```python
from build123d import *

# Parameters (mm, degrees)
BOSS_EXTRUDE1_DEPTH = 6.6


with BuildPart() as part:
    # Model → Boss-Extrude1 (new body)
    with BuildSketch(Plane.XY):
        with BuildLine():
            Line((72.9, 1.275), (72.9, -1.275))
            ThreePointArc((72.9, -1.275), (73.046446609, -1.628553391), (73.4, -1.775))
            Line((73.4, -1.775), (77.9, -1.775))
            Line((77.9, -1.775), (77.9, -3.36))
            ThreePointArc((77.9, -3.36), (78.046446609, -3.713553391), (78.4, -3.86))
            Line((78.4, -3.86), (82.4, -3.86))
            ThreePointArc((82.4, -3.86), (82.753553391, -3.713553391), (82.9, -3.36))
            Line((82.9, -3.36), (82.9, -1.775))
            Line((82.9, -1.775), (93.9, -1.775))
            Line((93.9, -1.775), (93.9, -27.3))
            Line((93.9, -27.3), (97.9, -27.3))
            ThreePointArc((97.9, -27.3), (99.667766953, -28.032233047), (100.4, -29.8))
            Line((100.4, -29.8), (100.4, -39.8))
            ThreePointArc((100.4, -39.8), (99.667766953, -41.567766953), (97.9, -42.3))
            Line((97.9, -42.3), (93.9, -42.3))
            Line((93.9, -42.3), (93.9, -55))
            Line((93.9, -55), (-93.9, -55))
            Line((-93.9, -55), (-93.9, -42.3))
            Line((-93.9, -42.3), (-97.9, -42.3))
            ThreePointArc((-97.9, -42.3), (-99.667766953, -41.567766953), (-100.4, -39.8))
            Line((-100.4, -39.8), (-100.4, -29.8))
            ThreePointArc((-100.4, -29.8), (-99.667766953, -28.032233047), (-97.9, -27.3))
            Line((-97.9, -27.3), (-93.9, -27.3))
            Line((-93.9, -27.3), (-93.9, -1.775))
            Line((-93.9, -1.775), (-82.9, -1.775))
            Line((-82.9, -1.775), (-82.9, -3.36))
            ThreePointArc((-82.9, -3.36), (-82.753553391, -3.713553391), (-82.4, -3.86))
            Line((-82.4, -3.86), (-78.4, -3.86))
            ThreePointArc((-78.4, -3.86), (-78.046446609, -3.713553391), (-77.9, -3.36))
            Line((-77.9, -3.36), (-77.9, -1.775))
            Line((-77.9, -1.775), (-73.4, -1.775))
            ThreePointArc((-73.4, -1.775), (-73.046446609, -1.628553391), (-72.9, -1.275))
            Line((-72.9, -1.275), (-72.9, 1.275))
            ThreePointArc((-72.9, 1.275), (-73.046446609, 1.628553391), (-73.4, 1.775))
            Line((-73.4, 1.775), (-77.9, 1.775))
            Line((-77.9, 1.775), (-77.9, 3.36))
            ThreePointArc((-77.9, 3.36), (-78.046446609, 3.713553391), (-78.4, 3.86))
            Line((-78.4, 3.86), (-82.4, 3.86))
            ThreePointArc((-82.4, 3.86), (-82.753553391, 3.713553391), (-82.9, 3.36))
            Line((-82.9, 3.36), (-82.9, 1.775))
            Line((-82.9, 1.775), (-93.9, 1.775))
            Line((-93.9, 1.775), (-93.9, 27.3))
            Line((-93.9, 27.3), (-97.9, 27.3))
            ThreePointArc((-97.9, 27.3), (-99.667766953, 28.032233047), (-100.4, 29.8))
            Line((-100.4, 29.8), (-100.4, 39.8))
            ThreePointArc((-100.4, 39.8), (-99.667766953, 41.567766953), (-97.9, 42.3))
            Line((-97.9, 42.3), (-93.9, 42.3))
            Line((-93.9, 42.3), (-93.9, 55))
            Line((-93.9, 55), (93.9, 55))
            Line((93.9, 55), (93.9, 42.3))
            Line((93.9, 42.3), (97.9, 42.3))
            ThreePointArc((97.9, 42.3), (99.667766953, 41.567766953), (100.4, 39.8))
            Line((100.4, 39.8), (100.4, 29.8))
            ThreePointArc((100.4, 29.8), (99.667766953, 28.032233047), (97.9, 27.3))
            Line((97.9, 27.3), (93.9, 27.3))
            Line((93.9, 27.3), (93.9, 1.775))
            Line((93.9, 1.775), (82.9, 1.775))
            Line((82.9, 1.775), (82.9, 3.36))
            ThreePointArc((82.9, 3.36), (82.753553391, 3.713553391), (82.4, 3.86))
            Line((82.4, 3.86), (78.4, 3.86))
            ThreePointArc((78.4, 3.86), (78.046446609, 3.713553391), (77.9, 3.36))
            Line((77.9, 3.36), (77.9, 1.775))
            Line((77.9, 1.775), (73.4, 1.775))
            ThreePointArc((73.4, 1.775), (73.046446609, 1.628553391), (72.9, 1.275))
        make_face()
        with BuildLine():
            Line((29.75, 34.05), (29.75, -29.45))
            ThreePointArc((29.75, -29.45), (26.25, -32.95), (22.75, -29.45))
            Line((22.75, -29.45), (22.75, 34.05))
            ThreePointArc((22.75, 34.05), (26.25, 37.55), (29.75, 34.05))
        make_face(mode=Mode.SUBTRACT)
        with BuildLine():
            Line((-29.75, 34.05), (-29.75, -29.45))
            ThreePointArc((-29.75, -29.45), (-26.25, -32.95), (-22.75, -29.45))
            Line((-22.75, -29.45), (-22.75, 34.05))
            ThreePointArc((-22.75, 34.05), (-26.25, 37.55), (-29.75, 34.05))
        make_face(mode=Mode.SUBTRACT)
        with BuildLine():
            Line((2.54, -29.45), (2.54, 34.05))
            ThreePointArc((2.54, 34.05), (0, 36.59), (-2.54, 34.05))
            Line((-2.54, 34.05), (-2.54, -29.45))
            ThreePointArc((-2.54, -29.45), (0, -31.99), (2.54, -29.45))
        make_face(mode=Mode.SUBTRACT)
        with BuildLine():
            Line((-39.75, -35), (-39.75, 35))
            ThreePointArc((-39.75, 35), (-42.678932188, 42.071067812), (-49.75, 45))
            Line((-49.75, 45), (-52.9, 45))
            ThreePointArc((-52.9, 45), (-59.971067812, 42.071067812), (-62.9, 35))
            Line((-62.9, 35), (-62.9, -35))
            ThreePointArc((-62.9, -35), (-59.971067812, -42.071067812), (-52.9, -45))
            Line((-52.9, -45), (-49.75, -45))
            ThreePointArc((-49.75, -45), (-42.678932188, -42.071067812), (-39.75, -35))
        make_face(mode=Mode.SUBTRACT)
        with BuildLine():
            Line((62.9, -35), (62.9, 35))
            ThreePointArc((62.9, 35), (59.971067812, 42.071067812), (52.9, 45))
            Line((52.9, 45), (49.75, 45))
            ThreePointArc((49.75, 45), (42.678932188, 42.071067812), (39.75, 35))
            Line((39.75, 35), (39.75, -35))
            ThreePointArc((39.75, -35), (42.678932188, -42.071067812), (49.75, -45))
            Line((49.75, -45), (52.9, -45))
            ThreePointArc((52.9, -45), (59.971067812, -42.071067812), (62.9, -35))
        make_face(mode=Mode.SUBTRACT)
    extrude(amount=BOSS_EXTRUDE1_DEPTH)


solid = part.part
```
Part model, mm, in its own coordinate system. A direction names the side the tool comes from. Round coordinates to 2 decimals unless told otherwise and drop trailing zeros. Loops run counter-clockwise (first coordinate to the right, second up) from the corner with the lowest first, then second, coordinate; pieces in that order, holes last.
Item 1: Drill centre lines: line 1 (X direction, y = 5.5, z = 1); line 2 (X direction, y = -35, z = 4.75); line 3 (X direction, y = -43, z = 2.75). Where is each one in solid material? Low to high.
Item 2: Drop flat-ended pins along their axis: P1, Ø3, axis at y = 0.5, z = 2.5, coming from the -X side; P2, Ø3.5, axis at y = -13, z = 3.5, coming from the +X side; P3, Ø3, axis at x = 95.5, z = 3, coming from the -Y side. Give the stop position or say it passes through.
Item 3: Mould opens along X. For faces 5 (the face through (96, 27.3, 3)), 6 (the face through (-26.33, -32.95, 3.25)), 7 (the face through (-93.9, 49, 3)) say: +X half, -X half, draft (parallel to the pull), parting line (faces both ways), or undercut.
Item 4: Cut at D-D, the plane z = 1. State how many separate pieces and enclosed holes the cut face has, then the cut area to 3 significant figures.
Item 5: Cut at B-B, the plane y = -8.5. Give the cut face in (x, z), then the cut area to 3 significant figures.
Item 6: Cut at A-A, the plane x = -87. Give the cut face in (y, z) (3 decimals), then the cut area to 3 significant figures.
Item 7: Cut at C-C, the plane x = 26.25. Give the cut face in (y, z).
Item 8: 3-axis set-ups, long thin cutter, end or side, ignore diameter. For faces 1 (the face through (-93.9, 14, 3)), 2 (the face through (93.9, 15, 3)), 3 (the face through (93.9, 49, 3)), 4 (the face through (22.75, 2, 3)): which of +Z, -Z, +X, -X, +Y, -Y reach the whole face in a straight line?
A:
1. line 1: x = -93.9 to -62.9, -39.75 to -29.75, -22.75 to -2.54, 2.54 to 22.75, 29.75 to 39.75, 62.9 to 93.9
1. line 2: x = -100.4 to -62.9, -39.75 to 39.75, 62.9 to 100.4
1. line 3: x = -93.9 to -58.9, -43.75 to 43.75, 58.9 to 93.9
2. P1: stops at x = -93.9
2. P2: stops at x = 93.9
2. P3: stops at y = -42.3
3. face 5: draft
3. face 6: undercut
3. face 7: -X half
4. separate pieces: 1
4. enclosed holes: 5
4. area: 15,500 mm2
5. outline: (-93.9, 0) - (-62.9, 0) - (-62.9, 6.6) - (-93.9, 6.6) - close; (-39.75, 0) - (-29.75, 0) - (-29.75, 6.6) - (-39.75, 6.6) - close; (-22.75, 0) - (-2.54, 0) - (-2.54, 6.6) - (-22.75, 6.6) - close; (2.54, 0) - (22.75, 0) - (22.75, 6.6) - (2.54, 6.6) - close; (29.75, 0) - (39.75, 0) - (39.75, 6.6) - (29.75, 6.6) - close; (62.9, 0) - (93.9, 0) - (93.9, 6.6) - (62.9, 6.6) - close
5. area: 808 mm2
6. outline: (-55, 0) - (-1.775, 0) - (-1.775, 6.6) - (-55, 6.6) - close; (1.775, 0) - (55, 0) - (55, 6.6) - (1.775, 6.6) - close
6. area: 703 mm2
7. outline: (-55, 0) - (-32.95, 0) - (-32.95, 6.6) - (-55, 6.6) - close; (37.55, 0) - (55, 0) - (55, 6.6) - (37.55, 6.6) - close
8. face 1: +Z, -Z, -X
8. face 2: +Z, -Z, +X
8. face 3: +Z, -Z, +X, +Y
8. face 4: +Z, -Z
